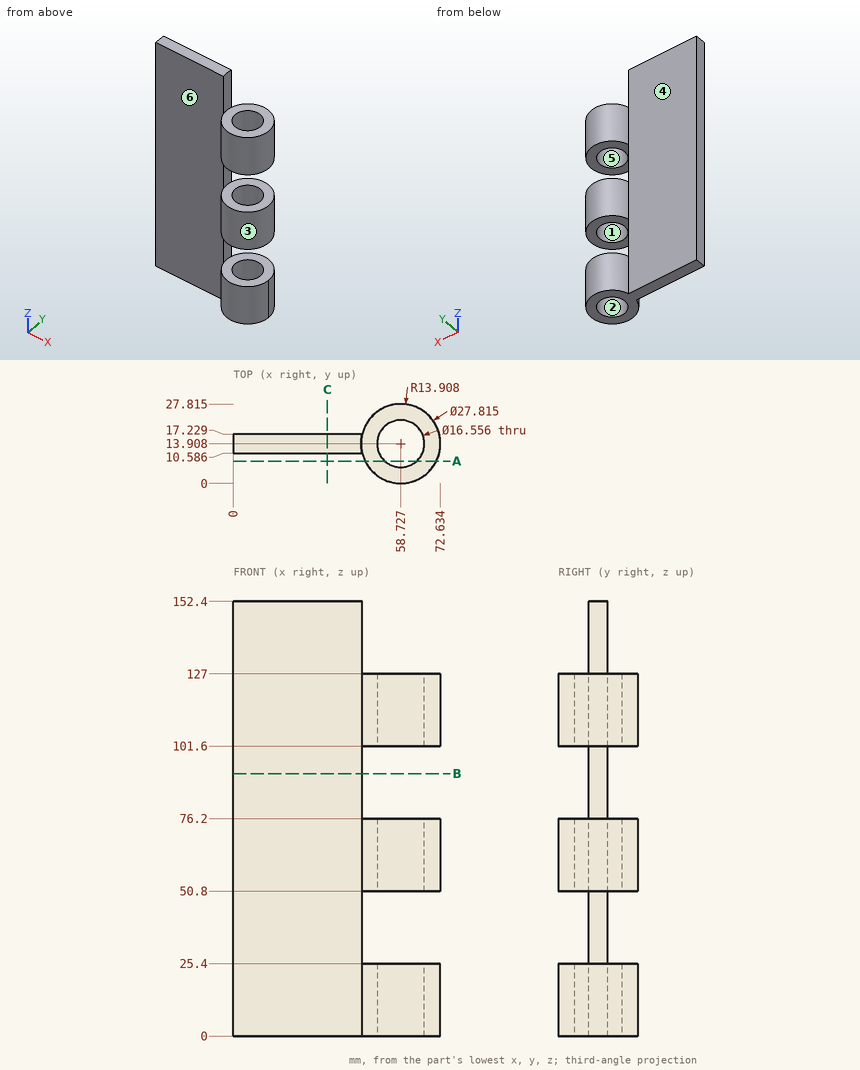
Drawing for the job (mm, zero at the part's lowest x, y, z). A direction names the side the tool comes from. Give positions to 0.01 mm unless a question says otherwise; leave off trailing zeros. Order: outer loops, then holes, each group sorted by start corner. A loop starts at its lowest first (then second) coordinate and runs counter-clockwise, first axis right, second up. Notation, with made-up numbers: M 77.5,49.25 L 96.5,49.25 A17 ccw 96.5,65.25 Z; hole C 76.5,-15.5 d5. An arc over 180 degrees is marked long. Write item = value, one per line. Start each with the question number.
(1) Slice it at C-C on x = 33. Write the cut outline in (y, z), plus the area to 3 significant figures.
(2) Slice it at B-B on z = 92. Write the cut outline in (x, y) (1 decimal).
(3) Which spindle directions (+Z, -Z, +X, -X, +Y, -Y) get a long thin tool onto all of the face, cutting with end or side? Do the marked faces 5 and 6. Say none if no direction does.
(4) Probe L1, parallel to Z at x = 68.5, y = 14.5; L2, parallel to X at y = 13.5, z = 110 (1 decimal); L3, parallel to X at y = 13.25, z = 133.5 (1 decimal). List the from-to ranges inside material, lowest first. Write a range as [from, to].
(5) Two-plate mould, pull along Y, no slides. Class the marked faces 1, 2, 3 and 4: released by +Y, released by -Y, zero draft, split by the parting line, or undercut.
(6) Pin check, flat tips, straight feed: pin 1 Ø5 at (x, z) = (24.5, 99.5) entering from -Y; pin 2 Ø1 at (y, z) = (7.5, 119.5) entering from -X (1 decimal); pin 3 Ø10 at (x, y) = (58.73, 13.91) entering from -Z; pin 4 Ø13.5 at (x, z) = (27, 41.5) entering from +Y. Stop position of each tip, or through.
(7) Slice it at A-A on y = 7.75. Write the cut outline in (x, z), plus the area to 3 significant figures.
Responses:
q1.outline = M 10.59,0 L 17.23,0 L 17.23,152.4 L 10.59,152.4 Z
q1.area = 1,010 mm2
q2.outline = M 0,10.6 L 45.2,10.6 A13.9 cw 45.2,17.2 L 0,17.2 Z
q3.face_5 = +Z, -Z
q3.face_6 = +Z, -Z, -X, -Y
q4.L1 = [0, 25.4], [50.8, 76.2], [101.6, 127]
q4.L2 = [0, 50.5], [67, 72.6]
q4.L3 = [0, 44.8]
q5.face_1 = undercut
q5.face_2 = undercut
q5.face_3 = split by the parting line
q5.face_4 = released by +Y
q6.pin_1 = 10.59
q6.pin_2 = 46.1
q6.pin_3 = through
q6.pin_4 = 17.23
q7.outline = M 46.26,0 L 53.19,0 L 53.19,25.4 L 46.26,25.4 Z; M 46.26,50.8 L 53.19,50.8 L 53.19,76.2 L 46.26,76.2 Z; M 46.26,101.6 L 53.19,101.6 L 53.19,127 L 46.26,127 Z; M 64.26,0 L 71.2,0 L 71.2,25.4 L 64.26,25.4 Z; M 64.26,50.8 L 71.2,50.8 L 71.2,76.2 L 64.26,76.2 Z; M 64.26,101.6 L 71.2,101.6 L 71.2,127 L 64.26,127 Z
q7.area = 1,060 mm2
